from build123d import *

# Parameters (mm, degrees)
SKETCH_1_R          = 8
EXTRUDE_1_DEPTH     = 6
SKETCH_2_R          = 6.870177757
EXTRUDE_2_DEPTH     = 8
CUT_EXTRUDE_START   = -8
CUT_EXTRUDE_1_DEPTH = 8
SKETCH_4_R          = 8
EXTRUDE_3_DEPTH     = 1
SKETCH_5_R          = 4
CUT_EXTRUDE_2_DEPTH = 19.788294228


with BuildPart() as part:
    # 草图1 → 凸台-拉伸1 (new body)
    with BuildSketch(Plane(origin=(0, 0, 0), x_dir=(1, 0, 0), z_dir=(0, 1, 0))):
        with Locations(Location((0, 0, 0), (0, 0, 270))):
            Circle(SKETCH_1_R)
    extrude(amount=EXTRUDE_1_DEPTH)

    # 草图2 → 凸台-拉伸2 (add)
    with BuildSketch(Plane(origin=(0, 6, 0), x_dir=(1, 0, 0), z_dir=(0, 1, 0))):
        with Locations(Location((0, 0, 0), (0, 0, 270))):
            Circle(SKETCH_2_R)
    extrude(amount=EXTRUDE_2_DEPTH)

    # 草图3 → 切除-拉伸1 (cut)
    with BuildSketch(Plane(origin=(0, 14, 0), x_dir=(1, 0, 0), z_dir=(0, 1, 0)).offset(CUT_EXTRUDE_START)):
        with BuildLine():
            Line((-0.70957594, 6.214911676), (-0.774732582, 6.785594468))
            Line((-0.774732582, 6.785594468), (-0.779326709, 6.825832718))
            ThreePointArc((-0.779326709, 6.825832718), (-1.074732582, 6.785594468), (-1.368114565, 6.732577883))
            Line((-1.368114565, 6.732577883), (-1.360049537, 6.69288937))
            Line((-1.360049537, 6.69288937), (-1.245666505, 6.130003271))
            Line((-1.245666505, 6.130003271), (-0.977621222, 6.172457473))
            Line((-0.977621222, 6.172457473), (-0.70957594, 6.214911676))
        make_face()
        with BuildLine():
            Line((1.245666505, 6.130003271), (1.360049537, 6.69288937))
            Line((1.360049537, 6.69288937), (1.368114565, 6.732577883))
            ThreePointArc((1.368114565, 6.732577883), (1.074732582, 6.785594468), (0.779326709, 6.825832718))
            Line((0.779326709, 6.825832718), (0.774732582, 6.785594468))
            Line((0.774732582, 6.785594468), (0.70957594, 6.214911676))
            Line((0.70957594, 6.214911676), (0.977621222, 6.172457473))
            Line((0.977621222, 6.172457473), (1.245666505, 6.130003271))
        make_face()
        with BuildLine():
            Line((3.078974433, 5.445047437), (3.361700531, 5.945037628))
            Line((3.361700531, 5.945037628), (3.381635254, 5.980291416))
            ThreePointArc((3.381635254, 5.980291416), (3.118995433, 6.121373204), (2.850482056, 6.250927488))
            Line((2.850482056, 6.250927488), (2.833678478, 6.214078302))
            Line((2.833678478, 6.214078302), (2.595360147, 5.691461223))
            Line((2.595360147, 5.691461223), (2.83716729, 5.56825433))
            Line((2.83716729, 5.56825433), (3.078974433, 5.445047437))
        make_face()
        with BuildLine():
            Line((4.610890891, 4.227092421), (5.034284855, 4.615244181))
            Line((5.034284855, 4.615244181), (5.064137923, 4.642612358))
            ThreePointArc((5.064137923, 4.642612358), (4.85794928, 4.85794928), (4.642612358, 5.064137923))
            Line((4.642612358, 5.064137923), (4.615244181, 5.034284855))
            Line((4.615244181, 5.034284855), (4.227092421, 4.610890891))
            Line((4.227092421, 4.610890891), (4.418991656, 4.418991656))
            Line((4.418991656, 4.418991656), (4.610890891, 4.227092421))
        make_face()
        with BuildLine():
            Line((5.691461223, 2.595360147), (6.214078302, 2.833678478))
            Line((6.214078302, 2.833678478), (6.250927488, 2.850482056))
            ThreePointArc((6.250927488, 2.850482056), (6.121373204, 3.118995433), (5.980291416, 3.381635254))
            Line((5.980291416, 3.381635254), (5.945037628, 3.361700531))
            Line((5.945037628, 3.361700531), (5.445047437, 3.078974433))
            Line((5.445047437, 3.078974433), (5.56825433, 2.83716729))
            Line((5.56825433, 2.83716729), (5.691461223, 2.595360147))
        make_face()
        with BuildLine():
            Line((6.214911676, 0.70957594), (6.785594468, 0.774732582))
            Line((6.785594468, 0.774732582), (6.825832718, 0.779326709))
            ThreePointArc((6.825832718, 0.779326709), (6.785594468, 1.074732582), (6.732577883, 1.368114565))
            Line((6.732577883, 1.368114565), (6.69288937, 1.360049537))
            Line((6.69288937, 1.360049537), (6.130003271, 1.245666505))
            Line((6.130003271, 1.245666505), (6.172457473, 0.977621222))
            Line((6.172457473, 0.977621222), (6.214911676, 0.70957594))
        make_face()
        with BuildLine():
            Line((6.130003271, -1.245666505), (6.69288937, -1.360049537))
            Line((6.69288937, -1.360049537), (6.732577883, -1.368114565))
            ThreePointArc((6.732577883, -1.368114565), (6.785594468, -1.074732582), (6.825832718, -0.779326709))
            Line((6.825832718, -0.779326709), (6.785594468, -0.774732582))
            Line((6.785594468, -0.774732582), (6.214911676, -0.70957594))
            Line((6.214911676, -0.70957594), (6.172457473, -0.977621222))
            Line((6.172457473, -0.977621222), (6.130003271, -1.245666505))
        make_face()
        with BuildLine():
            Line((5.445047437, -3.078974433), (5.945037628, -3.361700531))
            Line((5.945037628, -3.361700531), (5.980291416, -3.381635254))
            ThreePointArc((5.980291416, -3.381635254), (6.121373204, -3.118995433), (6.250927488, -2.850482056))
            Line((6.250927488, -2.850482056), (6.214078302, -2.833678478))
            Line((6.214078302, -2.833678478), (5.691461223, -2.595360147))
            Line((5.691461223, -2.595360147), (5.56825433, -2.83716729))
            Line((5.56825433, -2.83716729), (5.445047437, -3.078974433))
        make_face()
        with BuildLine():
            Line((4.227092421, -4.610890891), (4.615244181, -5.034284855))
            Line((4.615244181, -5.034284855), (4.642612358, -5.064137923))
            ThreePointArc((4.642612358, -5.064137923), (4.85794928, -4.85794928), (5.064137923, -4.642612358))
            Line((5.064137923, -4.642612358), (5.034284855, -4.615244181))
            Line((5.034284855, -4.615244181), (4.610890891, -4.227092421))
            Line((4.610890891, -4.227092421), (4.418991656, -4.418991656))
            Line((4.418991656, -4.418991656), (4.227092421, -4.610890891))
        make_face()
        with BuildLine():
            Line((2.595360147, -5.691461223), (2.833678478, -6.214078302))
            Line((2.833678478, -6.214078302), (2.850482056, -6.250927488))
            ThreePointArc((2.850482056, -6.250927488), (3.118995433, -6.121373204), (3.381635254, -5.980291416))
            Line((3.381635254, -5.980291416), (3.361700531, -5.945037628))
            Line((3.361700531, -5.945037628), (3.078974433, -5.445047437))
            Line((3.078974433, -5.445047437), (2.83716729, -5.56825433))
            Line((2.83716729, -5.56825433), (2.595360147, -5.691461223))
        make_face()
        with BuildLine():
            Line((0.70957594, -6.214911676), (0.774732582, -6.785594468))
            Line((0.774732582, -6.785594468), (0.779326709, -6.825832718))
            ThreePointArc((0.779326709, -6.825832718), (1.074732582, -6.785594468), (1.368114565, -6.732577883))
            Line((1.368114565, -6.732577883), (1.360049537, -6.69288937))
            Line((1.360049537, -6.69288937), (1.245666505, -6.130003271))
            Line((1.245666505, -6.130003271), (0.977621222, -6.172457473))
            Line((0.977621222, -6.172457473), (0.70957594, -6.214911676))
        make_face()
        with BuildLine():
            Line((-1.245666505, -6.130003271), (-1.360049537, -6.69288937))
            Line((-1.360049537, -6.69288937), (-1.368114565, -6.732577883))
            ThreePointArc((-1.368114565, -6.732577883), (-1.074732582, -6.785594468), (-0.779326709, -6.825832718))
            Line((-0.779326709, -6.825832718), (-0.774732582, -6.785594468))
            Line((-0.774732582, -6.785594468), (-0.70957594, -6.214911676))
            Line((-0.70957594, -6.214911676), (-0.977621222, -6.172457473))
            Line((-0.977621222, -6.172457473), (-1.245666505, -6.130003271))
        make_face()
        with BuildLine():
            Line((-3.078974433, -5.445047437), (-3.361700531, -5.945037628))
            Line((-3.361700531, -5.945037628), (-3.381635254, -5.980291416))
            ThreePointArc((-3.381635254, -5.980291416), (-3.118995433, -6.121373204), (-2.850482056, -6.250927488))
            Line((-2.850482056, -6.250927488), (-2.833678478, -6.214078302))
            Line((-2.833678478, -6.214078302), (-2.595360147, -5.691461223))
            Line((-2.595360147, -5.691461223), (-2.83716729, -5.56825433))
            Line((-2.83716729, -5.56825433), (-3.078974433, -5.445047437))
        make_face()
        with BuildLine():
            Line((-4.610890891, -4.227092421), (-5.034284855, -4.615244181))
            Line((-5.034284855, -4.615244181), (-5.064137923, -4.642612358))
            ThreePointArc((-5.064137923, -4.642612358), (-4.85794928, -4.85794928), (-4.642612358, -5.064137923))
            Line((-4.642612358, -5.064137923), (-4.615244181, -5.034284855))
            Line((-4.615244181, -5.034284855), (-4.227092421, -4.610890891))
            Line((-4.227092421, -4.610890891), (-4.418991656, -4.418991656))
            Line((-4.418991656, -4.418991656), (-4.610890891, -4.227092421))
        make_face()
        with BuildLine():
            Line((-5.691461223, -2.595360147), (-6.214078302, -2.833678478))
            Line((-6.214078302, -2.833678478), (-6.250927488, -2.850482056))
            ThreePointArc((-6.250927488, -2.850482056), (-6.121373204, -3.118995433), (-5.980291416, -3.381635254))
            Line((-5.980291416, -3.381635254), (-5.945037628, -3.361700531))
            Line((-5.945037628, -3.361700531), (-5.445047437, -3.078974433))
            Line((-5.445047437, -3.078974433), (-5.56825433, -2.83716729))
            Line((-5.56825433, -2.83716729), (-5.691461223, -2.595360147))
        make_face()
        with BuildLine():
            Line((-6.214911676, -0.70957594), (-6.785594468, -0.774732582))
            Line((-6.785594468, -0.774732582), (-6.825832718, -0.779326709))
            ThreePointArc((-6.825832718, -0.779326709), (-6.785594468, -1.074732582), (-6.732577883, -1.368114565))
            Line((-6.732577883, -1.368114565), (-6.69288937, -1.360049537))
            Line((-6.69288937, -1.360049537), (-6.130003271, -1.245666505))
            Line((-6.130003271, -1.245666505), (-6.172457473, -0.977621222))
            Line((-6.172457473, -0.977621222), (-6.214911676, -0.70957594))
        make_face()
        with BuildLine():
            Line((-6.130003271, 1.245666505), (-6.69288937, 1.360049537))
            Line((-6.69288937, 1.360049537), (-6.732577883, 1.368114565))
            ThreePointArc((-6.732577883, 1.368114565), (-6.785594468, 1.074732582), (-6.825832718, 0.779326709))
            Line((-6.825832718, 0.779326709), (-6.785594468, 0.774732582))
            Line((-6.785594468, 0.774732582), (-6.214911676, 0.70957594))
            Line((-6.214911676, 0.70957594), (-6.172457473, 0.977621222))
            Line((-6.172457473, 0.977621222), (-6.130003271, 1.245666505))
        make_face()
        with BuildLine():
            Line((-5.445047437, 3.078974433), (-5.945037628, 3.361700531))
            Line((-5.945037628, 3.361700531), (-5.980291416, 3.381635254))
            ThreePointArc((-5.980291416, 3.381635254), (-6.121373204, 3.118995433), (-6.250927488, 2.850482056))
            Line((-6.250927488, 2.850482056), (-6.214078302, 2.833678478))
            Line((-6.214078302, 2.833678478), (-5.691461223, 2.595360147))
            Line((-5.691461223, 2.595360147), (-5.56825433, 2.83716729))
            Line((-5.56825433, 2.83716729), (-5.445047437, 3.078974433))
        make_face()
        with BuildLine():
            Line((-4.227092421, 4.610890891), (-4.615244181, 5.034284855))
            Line((-4.615244181, 5.034284855), (-4.642612358, 5.064137923))
            ThreePointArc((-4.642612358, 5.064137923), (-4.85794928, 4.85794928), (-5.064137923, 4.642612358))
            Line((-5.064137923, 4.642612358), (-5.034284855, 4.615244181))
            Line((-5.034284855, 4.615244181), (-4.610890891, 4.227092421))
            Line((-4.610890891, 4.227092421), (-4.418991656, 4.418991656))
            Line((-4.418991656, 4.418991656), (-4.227092421, 4.610890891))
        make_face()
        with BuildLine():
            Line((-2.595360147, 5.691461223), (-2.833678478, 6.214078302))
            Line((-2.833678478, 6.214078302), (-2.850482056, 6.250927488))
            ThreePointArc((-2.850482056, 6.250927488), (-3.118995433, 6.121373204), (-3.381635254, 5.980291416))
            Line((-3.381635254, 5.980291416), (-3.361700531, 5.945037628))
            Line((-3.361700531, 5.945037628), (-3.078974433, 5.445047437))
            Line((-3.078974433, 5.445047437), (-2.83716729, 5.56825433))
            Line((-2.83716729, 5.56825433), (-2.595360147, 5.691461223))
        make_face()
    extrude(amount=CUT_EXTRUDE_1_DEPTH, mode=Mode.SUBTRACT)

    # 草图4 → 凸台-拉伸3 (add)
    with BuildSketch(Plane(origin=(0, 14, 0), x_dir=(1, 0, 0), z_dir=(0, 1, 0))):
        with Locations(Location((0, 0, 0), (0, 0, 270))):
            Circle(SKETCH_4_R)
    extrude(amount=EXTRUDE_3_DEPTH)

    # 草图5 → 切除-拉伸2 (cut, through all)
    with BuildSketch(Plane(origin=(0, 15, 0), x_dir=(1, 0, 0), z_dir=(0, 1, 0))):
        with Locations(Location((0, 0, 0), (0, 0, 270))):
            Circle(SKETCH_5_R)
    extrude(amount=-CUT_EXTRUDE_2_DEPTH, mode=Mode.SUBTRACT)


solid = part.part
Source: CAD feature listing. Evaluate the final solid. Frame: model axes, mm. A direction names the side the tool comes from. Give positions to 0.01 mm unless a question says otherwise; leave off trailing zeros. Write each loop counter-clockwise with the first axis right and the second up, starting at its lowest first coordinate (ties: lowest second). Pieces come first, ordered by that corner, then holes. Notation, with made-up numbers: M -25.75,-25 L 15.25,-25 A24 cw 15.25,12 Z; hole C -34,-22 d11. An arc over 180 degrees is marked long. Return JSON: item names as keys, results as strings. Group by question number.
1) Cut plane B-B, the plane z = 0. Output: boundary loops of the cut face in (x, y).
2) Cut plane C-C, the plane y = 4.75. Output: boundary loops of the cut face in (x, z).
3) Material intervals for line 1 along X through (y, z) = (6.5, 0); line 2 along X through (y, z) = (5, 0); line 3 along Y through (x, z) = (2, -6.75), sorted ascending. Write a range as [from, to].
4) Set-up query: faces 1 (the face through (6.87, 9.94, 0.01)), 2 (the face through (-6, 14, 3)), 3 (the face through (4.029, 9.944, 5.565)). Return all of +Z, -Z, +X, -X, +Y, -Y with unobstructed straight access to the full face (end or side cutting, diameter ignored); none if empty.
5) Pull-direction query (Z, two-part tool) for faces 4 (the face through (-2.11, 9.94, -6.54)), 5 (the face through (-3.905, 7.605, -0.867)), 6 (the face through (-0.01, 9.94, 6.87)); classes: pulls with the +Z half, pulls with the -Z half, needs draft (parallel to the pull), parting line crosses it, or undercut.
6) Cut plane A-A, the plane x = 0. Output: boundary loops of the cut face in (y, z).
7) Pin query (flat end, axial travel): P1, Ø3, axis at y = 2, z = 3, coming from the -X side; P2, Ø1, axis at y = 2.5, z = 3, coming from the -X side; P3, Ø3, axis at x = -2.5, y = 5, coming from the +Z side. Return the tip coordinate at first contact, or that it passes through.
Recorded:
{
 "1": {"outline": "M -8,0 L -4,0 L -4,15 L -8,15 L -8,14 L -6.87,14 L -6.87,6 L -8,6 Z; M 4,0 L 8,0 L 8,6 L 6.87,6 L 6.87,14 L 8,14 L 8,15 L 4,15 Z"},
 "2": {"outline": "C 0,0 d16; hole C 0,0 d8"},
 "3": {"line 1": "x = [-6.87, -4], [4, 6.87]", "line 2": "x = [-8, -4], [4, 8]", "line 3": "y = [0, 6], [14, 15]"},
 "4": {"face 1": "+X", "face 2": "none", "face 3": "+Z, +X"},
 "5": {"face 4": "pulls with the -Z half", "face 5": "undercut", "face 6": "pulls with the +Z half"},
 "6": {"outline": "M 0,-8 L 6,-8 L 6,-6.87 L 14,-6.87 L 14,-8 L 15,-8 L 15,-4 L 0,-4 Z; M 0,4 L 15,4 L 15,8 L 14,8 L 14,6.87 L 6,6.87 L 6,8 L 0,8 Z"},
 "7": {"P1": "stops at x = -7.86", "P2": "stops at x = -7.6", "P3": "stops at z = 7.94"}
}
